Model file for the job. Use its own axes, mm. A direction names the side the tool comes from. Give positions to 0.01 mm unless a question says otherwise; leave off trailing zeros. Loops run counter-clockwise (first coordinate to the right, second up) from the corner with the lowest first, then second, coordinate; pieces in that order, holes last. Notation, with made-up numbers: (27.25, -0.75) - (46.25, -0.75) arc R7 ccw to (46.25, 10.25) - close; hole circle Ø11 at (4.5, -26.75). An arc over 180 degrees is marked (long way). Answer as CSV lines item,"result". Start each with the question number.
Item 1: Drill centre lines: L1, parallel to X at y = 9, z = 525; L2, parallel to Z at x = -825, y = -3; L3, parallel to Z at x = -825, y = 7. Where is each one in solid material? Low to high. Write a range as from..to.
Item 2: Pull direction X, two halves, no side cores. Call faces 1 (the cylindrical face through (-614.766, 798.417, -6.93)), 2 (the flat face through (4, 900, -7)), 3 (the cylindrical face through (609.437, 807.769, -7)), 4 (the cylindrical face through (-868.058, 452.387, 6.93)): pulls with the +X half, pulls with the -X half, needs draft (parallel to the pull), parting line crosses it, or undercut.
Item 3: Tool access for faces 5 (the flat face through (-13, 752, 495)), 6 (the flat face through (-824, 20, 514)), 7 (the flat face through (900, 173, -8)): list every direction of +Z, -Z, +X, -X, +Y, -Y with a clear straight run to the whole face (end or side of a thin tool).
Item 4: Saw through at A-A on z = -378. Give the cut face in (x, y), plus the area to 3 significant figures.
Item 5: Saw through at B-B on y = 71. Give the cut face in (x, z), plus the area to 3 significant figures.
Item 6: Pin check, flat tips, straight feed: pin 1 (12 mm diameter, centred on x = -825, z = 525, fed in from -Y); pin 2 (2 mm diameter, centred on x = -45, y = 195, fed in from +Z); pin 3 (4 mm diameter, centred on x = -234, y = 411, fed in from -Z); pin 4 (4 mm diameter, centred on x = -423.5, z = 376.5, fed in from +Y). Stop position of each tip, or through.
Item 7: Saw through at C-C on x = -707.5. Give the cut face in (y, z).
Autodesk Inventor part; units mm, degrees
ref_plane "YZ Plane" through (0, 0, 0) normal (1, 0, 0) x (0, 1, 0)
ref_plane "XZ Plane" through (0, 0, 0) normal (0, 1, 0) x (-1, 0, 0)
ref_plane "XY Plane" through (0, 0, 0) normal (0, 0, 1) x (1, 0, 0)
sketch "Sketch1" plane through (0, 0, 0) normal (0, 0, 1) x (1, 0, 0)
  line L0 (-900, 0) -> (900, 0)
  line L1 (900, 0) -> (900, 900)
  line L2 (900, 900) -> (-900, 900)
  line L3 (-900, 900) -> (-900, 0)
  line L4 (0, 900) -> (0, 0) construction
  dimension "d0" = 900
  dimension "length" = 1800
extrude "Extrusion1" add sketch "Sketch1" along normal mid plane 1000
sketch "Sketch2" plane through (0, 0, 500) normal (0, 0, 1) x (1, 0, 0)
  line L0 (-900, 900) -> (-900, 0)
  arc A0 (-550, 900) -> (-900, 350) centre (-17.254, 174.6162) ccw
  line L1 (900, 900) -> (-900, 900)
  line L2 (-900, 350) -> (-900, 900)
  line L3 (-900, 900) -> (-550, 900)
  point P0 (0, 0)
  dimension "d5" = 900
  dimension "d6" = 550
  dimension "d7" = 350
extrude "Extrusion2" cut sketch "Sketch2" against normal blind 1000
mirror "Mirror1" about plane through (0, 0, 0) normal (1, 0, 0) of "Extrusion2"
fillet "Fillet1" radius 600 2 edges at (-550, 900, 0) (550, 900, 0)
sketch "Sketch3" plane through (0, 0, 500) normal (0, 0, 1) x (1, 0, 0)
  arc A0 (-289.7955, 900) -> (-834.8786, 550.7676) centre (-289.7955, 300) ccw
  line L0 (289.7955, 900) -> (-289.7955, 900)
  arc A1 (834.8786, 550.7676) -> (289.7955, 900) centre (289.7955, 300) ccw
  arc A2 (-289.7955, 750) -> (-625.2057, 600) centre (-289.7955, 300) ccw
  line L1 (-289.7955, 750) -> (289.7955, 750)
  arc A3 (625.2057, 600) -> (289.7955, 750) centre (289.7955, 300) ccw
  line L2 (-625.2057, 600) -> (-625.2057, 0)
  line L3 (900, 0) -> (-900, 0)
  line L4 (625.2057, 600) -> (625.2057, 0)
  line L5 (625.2057, 0) -> (-625.2057, 0)
  point P0 (0, 0)
  point P1 (625.2057, 0)
  dimension "d11" = 150
  dimension "d12" = 600
shell "Shell2" thickness 5 removed faces 1 at (300, 0, 166.6667)
extrude "Extrusion3" cut sketch "Sketch3" against normal blind 10
fillet "Fillet2" radius 600 2 edges at (-625.2057, 600, 497.5) (625.2057, 600, 497.5)
sketch "Sketch4" plane through (-900, 0, -500) normal (0, -1, 0) x (1, 0, 0)
  line L0 (1525.2057, 1000) -> (1800, 1000)
  line L1 (0, 0) -> (1800, 0)
  line L2 (1800, 0) -> (1800, 1000)
  line L3 (1800, 1000) -> (0, 1000)
  line L4 (0, 1000) -> (0, 0)
  point P0 (900, 500)
extrude "Extrusion4" add sketch "Sketch4" along normal blind 10
sketch "Sketch5" plane through (0, 0, 500) normal (0, 0, 1) x (1, 0, 0)
  line L0 (-900, -10) -> (900, -10)
  line L1 (-900, -10) -> (-750, -10)
  line L2 (-750, -10) -> (-750, 20)
  line L3 (-750, 20) -> (-900, 20)
  line L4 (-900, 20) -> (-900, -10)
  line L5 (900, -10) -> (750, -10)
  line L6 (750, -10) -> (750, 20)
  line L7 (750, 20) -> (900, 20)
  line L8 (900, 20) -> (900, -10)
  point P0 (0, 0)
  dimension "d19" = 30
  dimension "d20" = 150
extrude "Extrusion5" add sketch "Sketch5" along normal blind 50
sketch "Sketch6" plane through (-900, 20, 500) normal (0, 1, 0) x (1, 0, 0)
  circle A0 centre (75, -25) radius 10
  circle A1 centre (1725, -25) radius 10
  line L0 (75, -25) -> (1725, -25) construction
  line L1 (1800, -50) -> (1650, -50) construction
  line L2 (1650, 0) -> (1650, -50) construction
  line L3 (0, 0) -> (0, -50) construction
  line L4 (75, -25) -> (0, -25) construction
  line L5 (1725, -25) -> (1800, -25) construction
  line L6 (1800, 1000) -> (1800, -50) construction
  point P0 (900, 500)
  dimension "d25" = 20
  dimension "d31" = 1650
  dimension "d32" = 75
extrude "Extrusion6" cut sketch "Sketch6" against normal blind 30
mirror "Mirror2" about plane through (0, 0, 0) normal (0, 0, 1) of "Extrusion6", "Extrusion5"
ref_plane "Work Plane1" through (0, 0, 0) normal (1, 0, 0) x (0, 1, 0)
equation "\"d0\" = 0.5 * length"
equation "\"d5\" = 0.5 * length"
equation "\"d11\" = 0.0833333 * length"
equation "\"d12\" = 0.333333 * length"
equation "\"d13\" = 0.00277778 * length"
equation "\"d14\" = 0.00555556 * length"
equation "\"d17\" = 0.00555556 * length"
equation "\"d19\" = 0.0166667 * length"
equation "\"d20\" = 0.0833333 * length"
equation "\"d23\" = 0.0277778 * length"
equation "\"d25\" = 0.02 * d2"
equation "\"d32\" = 0.0416667 * length"
equation "\"d29\" = 0.0166667 * length"
properties part number "COVER, updated"
Responses:
1,L1,"-900..-835, -815..-750, 750..815, 835..900"
1,L2,"-550..-535, -515..515, 535..550"
1,L3,"-550..-535, -515..-495, 495..515, 535..550"
2,face 1,"undercut"
2,face 2,"needs draft"
2,face 3,"pulls with the +X half"
2,face 4,"undercut"
3,face 5,"none"
3,face 6,"+Z, +X, -X, +Y"
3,face 7,"+Z, -Z, +X, +Y, -Y"
4,outline,"(-900, -10) - (900, -10) - (900, 350) arc R900 ccw to (834.88, 550.77) arc R600 ccw to (289.8, 900) - (-289.8, 900) arc R600 ccw to (-834.88, 550.77) arc R900 ccw to (-900, 350) - close; hole (-895, 0) - (895, 0) - (895, 349.51) arc R895 ccw to (830.34, 548.68) arc R595 ccw to (289.8, 895) - (-289.8, 895) arc R595 ccw to (-830.34, 548.68) arc R895 ccw to (-895, 349.51) - close"
4,area,"33,300 mm2"
5,outline,"(-900, -500) - (900, -500) - (900, 500) - (625.21, 500) - (625.21, 495) - (895, 495) - (895, -495) - (-895, -495) - (-895, 495) - (-625.21, 495) - (-625.21, 500) - (-900, 500) - close"
5,area,"21,600 mm2"
6,pin 1,"through"
6,pin 2,"z = -495"
6,pin 3,"z = -500"
6,pin 4,"y = 885.37"
7,outline,"(-10, -500) - (730.72, -500) - (730.72, 500) - (-10, 500) - close; hole (0, -495) - (723.73, -495) - (723.73, 495) - (0, 495) - close"
